Here's how the part is built. I have some questions about the finished solid (model axes, mm). Give positions to 0.01 mm unless a question says otherwise; leave off trailing zeros. Order: outer loops, then holes, each group sorted by start corner. A loop starts at its lowest first (then second) coordinate and runs counter-clockwise, first axis right, second up. Notation, with made-up numbers: (-16, 85.25) -> (-1, 85.25) arc R13 ccw to (-1, 104.25) -> close; hole circle Ø11 at (42, 35.25). An arc over 180 degrees is marked (long way). Write each question's results on one line, items separated by ' | '. Start each with the question number.
Q1. Imagine slicing it at D-D, the plane z = 0.55. Please give me the cut outline in (x, y).
Q2. Imagine slicing it at C-C, the plane x = -17.5. Please give me the cut outline in (y, z), then the cut area to 3 significant figures.
Q3. Imagine slicing it at B-B, the plane y = 9.5. Please give me the cut outline in (x, z).
Q4. I need wall thicknesses on line 1 along X through (y, z) = (2, 1.9); line 2 along Y through (x, z) = (22.5, 1.65); line 3 along Y through (x, z) = (-17.5, 1.4). Which ranges of each line are inside material? Lowest first, please. Write a range as [from, to].
Q5. Imagine slicing it at A-A, the plane x = 14.5. Please give me the cut outline in (y, z), then the cut area to 3 significant figures.
Q6. I'm going to push a flat-ended pin straight in: pin 1 (3 mm diameter, centred on x = -26.5, y = 2.11, fed in from -Z). Where does the tip first touch, or does it pass through?
Solid Edge part; units mm, degrees
sketch "Sketch1" plane through (0, 0, 0) normal (0, 0, 1) x (1, 0, 0)
  line L0 (32.5, -16) -> (-32.5, -16)
  line L1 (-32.5, -16) -> (-32.5, 16)
  line L2 (-32.5, 16) -> (32.5, 16)
  line L3 (32.5, 16) -> (32.5, -16)
  dimension "D1" = 32.5
  dimension "D2" = 32.5
extrude "Protrusion1" add sketch "Sketch1" along normal blind 3
hole "Hole_1" at (7.5, 2.1097, 3) direction (0, 0, -1) diameter 6 end through all
hole "Hole_2" at (14.5, -13.3903, 3) direction (0, 0, -1) diameter 3.2 end through all
hole "Hole1" at (1.0766, 9.8597, 3) direction (0, 0, -1) diameter 3.2 end through all
hole "Hole2" at (27.9234, 9.8597, 3) direction (0, 0, -1) diameter 3.2 end through all
hole "Hole3" at (22.5, -9.1903, 3) direction (0, 0, -1) diameter 3.2 end through all
hole "Hole_6" at (-17.5, 2.1097, 0) direction (0, 0, 1) diameter 9 end through all
hole "Hole_7" at (-26.5, 2.1097, 0) direction (0, 0, 1) diameter 3.2 end through all
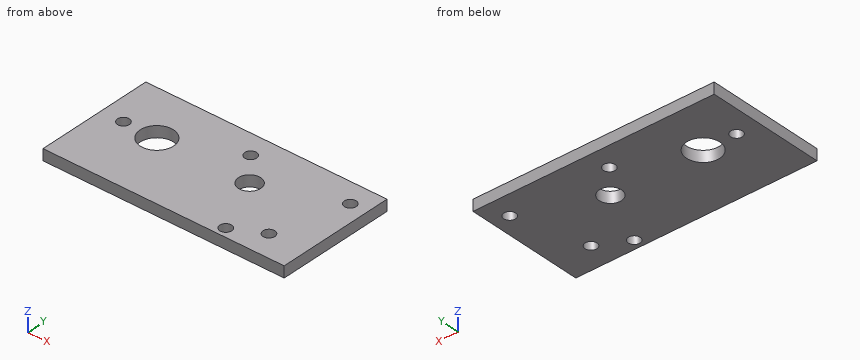
Geometry check:
1) outline: (-32.5, -16) -> (32.5, -16) -> (32.5, 16) -> (-32.5, 16) -> close; hole circle Ø3.2 at (-26.5, 2.11); hole circle Ø9 at (-17.5, 2.11); hole circle Ø3.2 at (1.08, 9.86); hole circle Ø6 at (7.5, 2.11); hole circle Ø3.2 at (14.5, -13.39); hole circle Ø3.2 at (22.5, -9.19); hole circle Ø3.2 at (27.92, 9.86)
2) outline: (-16, 0) -> (-2.39, 0) -> (-2.39, 3) -> (-16, 3) -> close; (6.61, 0) -> (16, 0) -> (16, 3) -> (6.61, 3) -> close | area: 69.0 mm²
3) outline: (-32.5, 0) -> (-0.48, 0) -> (-0.48, 3) -> (-32.5, 3) -> close; (2.64, 0) -> (26.36, 0) -> (26.36, 3) -> (2.64, 3) -> close; (29.48, 0) -> (32.5, 0) -> (32.5, 3) -> (29.48, 3) -> close
4) line 1: [-32.5, -28.1], [-24.9, -22], [-13, 4.5], [10.5, 32.5] | line 2: [-16, -10.79], [-7.59, 16] | line 3: [-16, -2.39], [6.61, 16]
5) outline: (-16, 0) -> (-14.99, 0) -> (-14.99, 3) -> (-16, 3) -> close; (-11.79, 0) -> (16, 0) -> (16, 3) -> (-11.79, 3) -> close | area: 86.4 mm²
6) pin 1: through
